Geometry: final body of the model. Coordinates: model frame, mm. Give positions to 0.01 mm unless a question says otherwise; leave off trailing zeros. Write each loop counter-clockwise with the first axis right and the second up, starting at its lowest first coordinate (ties: lowest second). Pieces come first, ordered by that corner, then holes.
Q1. Cut plane A-A on y = 0.9. Return the cut outline in (x, z).
Q2. Line query: L1, parallel to X at y = 0.35, z = -45.5; L2, parallel to X at y = 1.2, z = -51.5; L3, parallel to X at y = 1.25, z = -58. Output: solid intervals per line, ascending.
Q3. Cut plane C-C on x = 68. Return the cut outline in (y, z), plus the area to 3 significant figures.
Q4. Pin query (flat end, axial travel): pin 1 (0.5 mm diameter, centred on y = 0.5, z = -55, fed in from -X); pin 2 (0.5 mm diameter, centred on y = 0.5, z = -67.5, fed in from -X); pin 3 (0.8 mm diameter, centred on x = -87, y = 1, fed in from -Z). Return the tip coordinate at first contact, or that it passes through.
Q5. Cut plane B-B on x = 37.5. Return the cut outline in (y, z).
```python
from build123d import *

# Parameters (mm, degrees)
SKETCH1_W           = 224.63125
SKETCH1_H           = 143.66875
BOSS_EXTRUDE1_DEPTH = 1.524
CUT_EXTRUDE1_REACH  = 135.332
SKETCH2_W           = 157.95625
SKETCH2_H           = 34.13125
CHAMFER1_SIZE       = 3.175
SKETCH3_W           = 25.4
SKETCH3_H           = 12.7
BOSS_EXTRUDE2_DEPTH = 1.524
CUT_EXTRUDE2_REACH  = 135.332
CUT_EXTRUDE3_REACH  = 135.332
SKETCH5_W           = 6.35
SKETCH5_H           = 17.4625
CHAMFER2_SIZE       = 3.175
CUT_EXTRUDE4_REACH  = 135.332
SKETCH6_W           = 7.9375
SKETCH6_H           = 4.7625
SKETCH6_H_2         = 7.9375
CHAMFER3_SIZE       = 3.175


with BuildPart() as part:
    # Sketch1 → Boss-Extrude1 (new body)
    with BuildSketch(Plane(origin=(0, 0, 0), x_dir=(1, 0, 0), z_dir=(0, 1, 0))):
        Rectangle(SKETCH1_W, SKETCH1_H)
    extrude(amount=BOSS_EXTRUDE1_DEPTH)

    # Sketch2 → Cut-Extrude1 (cut, up to next)
    with BuildSketch(Plane(origin=(0, 1.524, 0), x_dir=(1, 0, 0), z_dir=(0, 1, 0)), mode=Mode.PRIVATE) as cut_extrude1_sk1:
        with Locations((0, 54.76875)):
            Rectangle(SKETCH2_W, SKETCH2_H)
    cut_extrude1_tool1 = extrude(cut_extrude1_sk1.sketch, amount=-CUT_EXTRUDE1_REACH, mode=Mode.PRIVATE) & part.part
    add(cut_extrude1_tool1.solids().sort_by_distance((0, 1.524, -54.76875))[0], mode=Mode.SUBTRACT)

    # Chamfer1
    chamfer1_edges = [part.edges().sort_by_distance(p)[0] for p in [
        (-78.978125, 0.762, -37.703125),
        (78.978125, 0.762, -37.703125),
    ]]
    chamfer(chamfer1_edges, length=CHAMFER1_SIZE)

    # Sketch3 → Boss-Extrude2 (add)
    with BuildSketch(Plane(origin=(0, 1.524, 0), x_dir=(1, 0, 0), z_dir=(0, 1, 0))):
        with Locations((31.353125, 44.053125)):
            Rectangle(SKETCH3_W, SKETCH3_H)
    extrude(amount=-BOSS_EXTRUDE2_DEPTH)

    # Sketch4 → Cut-Extrude2 (cut, up to next)
    with BuildSketch(Plane(origin=(0, 1.524, 0), x_dir=(1, 0, 0), z_dir=(0, 1, 0)), mode=Mode.PRIVATE) as cut_extrude2_sk1:
        Polygon((-78.978125, 56.753125), (-94.853125, 56.753125), (-94.853125, 47.228125), (-112.315625, 47.228125), (-112.315625, 71.834375), (-78.978125, 71.834375), align=None)
    cut_extrude2_tool1 = extrude(cut_extrude2_sk1.sketch, amount=-CUT_EXTRUDE2_REACH, mode=Mode.PRIVATE) & part.part
    add(cut_extrude2_tool1.solids().sort_by_distance((-97.620039, 1.524, -61.235346))[0], mode=Mode.SUBTRACT)

    # Sketch5 → Cut-Extrude3 (cut, up to next)
    with BuildSketch(Plane(origin=(0, 1.524, 0), x_dir=(1, 0, 0), z_dir=(0, 1, 0)), mode=Mode.PRIVATE) as cut_extrude3_sk1:
        with Locations((82.153125, 63.103125)):
            Rectangle(SKETCH5_W, SKETCH5_H)
    cut_extrude3_tool1 = extrude(cut_extrude3_sk1.sketch, amount=-CUT_EXTRUDE3_REACH, mode=Mode.PRIVATE) & part.part
    add(cut_extrude3_tool1.solids().sort_by_distance((82.153125, 1.524, -63.103125))[0], mode=Mode.SUBTRACT)

    # Chamfer2
    chamfer2_edges = [part.edges().sort_by_distance(p)[0] for p in [
        (-94.853125, 0.762, -47.228125),
        (85.328125, 0.762, -54.371875),
    ]]
    chamfer(chamfer2_edges, length=CHAMFER2_SIZE)

    # Sketch6 → Cut-Extrude4 (cut, up to next)
    with BuildSketch(Plane(origin=(0, 1.524, 0), x_dir=(1, 0, 0), z_dir=(0, 1, 0)), mode=Mode.PRIVATE) as cut_extrude4_sk1:
        with Locations((-108.346875, -69.453125)):
            Rectangle(SKETCH6_W, SKETCH6_H)
    cut_extrude4_tool1 = extrude(cut_extrude4_sk1.sketch, amount=-CUT_EXTRUDE4_REACH, mode=Mode.PRIVATE) & part.part
    # Sketch6 → Cut-Extrude4 (cut, up to next)
    with BuildSketch(Plane(origin=(0, 1.524, 0), x_dir=(1, 0, 0), z_dir=(0, 1, 0)), mode=Mode.PRIVATE) as cut_extrude4_sk2:
        with Locations((108.346875, -67.865625)):
            Rectangle(SKETCH6_W, SKETCH6_H_2)
    cut_extrude4_tool2 = extrude(cut_extrude4_sk2.sketch, amount=-CUT_EXTRUDE4_REACH, mode=Mode.PRIVATE) & part.part
    add(cut_extrude4_tool1.solids().sort_by_distance((-108.346875, 1.524, 69.453125))[0], mode=Mode.SUBTRACT)
    add(cut_extrude4_tool2.solids().sort_by_distance((108.346875, 1.524, 67.865625))[0], mode=Mode.SUBTRACT)

    # Chamfer3
    chamfer3_edges = [part.edges().sort_by_distance(p)[0] for p in [
        (112.315625, 0.762, 63.896875),
    ]]
    chamfer(chamfer3_edges, length=CHAMFER3_SIZE)


solid = part.part
```
Data:
1. outline: (-112.32, -47.23) - (-98.03, -47.23) - (-94.85, -50.4) - (-94.85, -56.75) - (-78.98, -56.75) - (-78.98, -40.88) - (-75.8, -37.7) - (18.65, -37.7) - (18.65, -50.4) - (44.05, -50.4) - (44.05, -37.7) - (75.8, -37.7) - (78.98, -40.88) - (78.98, -54.37) - (82.15, -54.37) - (85.33, -57.55) - (85.33, -71.83) - (112.32, -71.83) - (112.32, 60.72) - (109.14, 63.9) - (104.38, 63.9) - (104.38, 71.83) - (-104.38, 71.83) - (-104.38, 67.07) - (-112.32, 67.07) - close
2. L1: x = -112.32 to -78.98, 18.65 to 44.05, 78.98 to 112.32
2. L2: x = -94.85 to -78.98, 78.98 to 112.32
2. L3: x = 85.33 to 112.32
3. outline: (0, -37.7) - (1.52, -37.7) - (1.52, 71.83) - (0, 71.83) - close
3. area: 167 mm2
4. pin 1: stops at x = -94.85
4. pin 2: stops at x = 85.33
4. pin 3: stops at z = -56.75
5. outline: (0, -50.4) - (1.52, -50.4) - (1.52, 71.83) - (0, 71.83) - close
